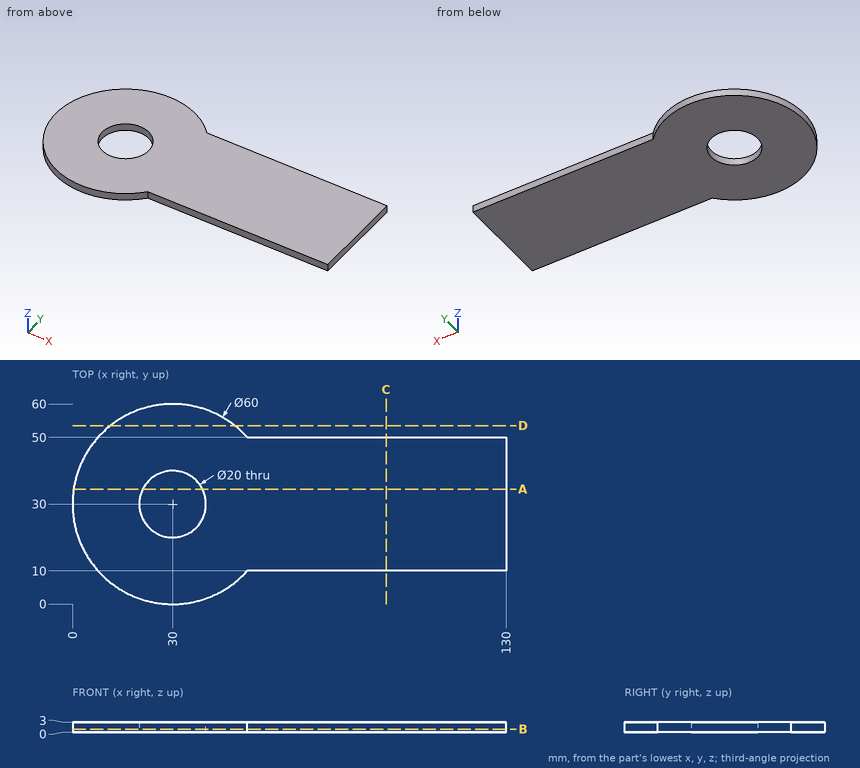
For this review, use the dimensioned drawing (mm, ordinates from the lowest corner) and the shaded views. Coordinates: 2 decimals unless noted, no trailing zeros. Write each loop counter-clockwise with the first axis right and the second up, starting at its lowest first coordinate (ties: lowest second). Pieces come first, ordered by that corner, then holes. Notation, with made-up numbers: (44, 76.25) - (52, 76.25) arc R32 cw to (52, 108.25) - close; hole circle Ø7 at (34.25, 69.25). An arc over 180 degrees is marked (long way). Answer in a Markdown table with one row per item. Add a question column.
Q1. Clearance check with flat-ended pins moving along their axes: pin 1 (0.9 mm diameter, centred on x = 94.5, z = 1, fed in from +Y); pin 2 (1 mm diameter, centred on y = 26, z = 1, fed in from -X); pin 3 (1.5 mm diameter, centred on x = 72.5, z = 2, fed in from -Y); pin 4 (1 mm diameter, centred on x = 105.5, y = 8, fed in from -Z). State where each tip first meets the part, or that it passes through.
Q2. Consider section C-C on x = 94. Give the boundary of the cut face in (y, z).
Q3. Consider section D-D on y = 53.5. Give the boundary of the cut face in (x, z).
Q4. Consider section B-B on z = 0.9. Give the boundary of the cut face in (x, y).
Q5. Consider section A-A on y = 34.5. Give the boundary of the cut face in (x, z).
Q6. To check wall thickness, follow line 1 along X through (y, z) = (23.5, 1.25); line 2 along Y through (x, z) = (34, 1.15); line 3 along Y through (x, z) = (82, 2.1). State the ranges of each line that lie inside material, in increasing order. Write a range as from..to.
Answers below:
| question | item | result |
|---|---|---|
| 1 | pin 1 | y = 50 |
| 1 | pin 2 | x = 0.2 |
| 1 | pin 3 | y = 10 |
| 1 | pin 4 | through |
| 2 | outline | (10, 0) - (50, 0) - (50, 3) - (10, 3) - close |
| 3 | outline | (11.35, 0) - (48.65, 0) - (48.65, 3) - (11.35, 3) - close |
| 4 | outline | (52.36, 10) - (130, 10) - (130, 50) - (52.36, 50) arc R30 ccw (long way) to start; hole circle Ø20 at (30, 30) |
| 5 | outline | (0.34, 0) - (21.07, 0) - (21.07, 3) - (0.34, 3) - close; (38.93, 0) - (130, 0) - (130, 3) - (38.93, 3) - close |
| 6 | line 1 | 0.71..22.4, 37.6..130 |
| 6 | line 2 | 0.27..20.83, 39.17..59.73 |
| 6 | line 3 | 10..50 |
